```python
from build123d import *

# Parameters (mm, degrees)
ESQUISSE2_R             = 1.5
ENL_V_MAT_EXTRU_1_DEPTH = 21.928449536
ESQUISSE3_W             = 17.74823935
ESQUISSE3_H             = 7.774498086
ENL_V_MAT_EXTRU_2_DEPTH = 20.052558883
CONG_1_R                = 1


with BuildPart() as part:
    # Esquisse1 → R_volution1 (revolve)
    with BuildSketch(Plane.XY, mode=Mode.PRIVATE) as r_volution1_sk:
        Polygon((4, 0), (4, 15), (5, 15), (5, 4), (11, 4), (11, 1), (5, 1), (5, 0), align=None)
    revolve(r_volution1_sk.sketch.rotate(Axis((0, 0, 0), (0, 1, 0)), 90), axis=Axis((0, 0, 0), (0, 1, 0)))

    # Esquisse2 → Enl_v. mat.-Extru.1 (cut, through all)
    with BuildSketch(Plane.XZ.offset(-1)):
        with Locations(Location((7.778174593, 0, 0), (0, 0, 270))):
            Circle(ESQUISSE2_R)
        with Locations(Location((0, -7.778174593, 0), (0, 0, 270))):
            Circle(ESQUISSE2_R)
        with Locations(Location((-7.778174593, 0, 0), (0, 0, 270))):
            Circle(ESQUISSE2_R)
        with Locations(Location((0, 7.778174593, 0), (0, 0, 270))):
            Circle(ESQUISSE2_R)
    extrude(amount=-ENL_V_MAT_EXTRU_1_DEPTH, mode=Mode.SUBTRACT)

    # Esquisse3 → Enl_v. mat.-Extru.2 (cut, through all)
    with BuildSketch(Plane(origin=(0, 4, 0), x_dir=(1, 0, 0), z_dir=(0, 1, 0))):
        with Locations((0, 10.387249043)):
            Rectangle(ESQUISSE3_W, ESQUISSE3_H)
    extrude(amount=-ENL_V_MAT_EXTRU_2_DEPTH, mode=Mode.SUBTRACT)

    # Cong_1
    # the kernel refuses this fillet: 1 mm, written as the material it takes off along each edge
    with BuildSketch(Plane(origin=(11.374119675, 1, -6.5), x_dir=(0, 0, 1), z_dir=(-1, 0, 0)), Plane(origin=(1.714971523, 1, -6.5), x_dir=(0, 0, 1), z_dir=(-1, 0, 0))) as cong_1_piece_1:
        with BuildLine():
            CenterArc((CONG_1_R, CONG_1_R), CONG_1_R, 180, 90)
            Line((0, CONG_1_R), (0, 0))
            Line((0, 0), (CONG_1_R, 0))
        make_face()
    extrude(amount=13.089091198, mode=Mode.SUBTRACT)
    with BuildSketch(Plane(origin=(1.714971523, 4, -6.5), x_dir=(0, 0, 1), z_dir=(-1, 0, 0)), Plane(origin=(11.374119675, 4, -6.5), x_dir=(0, 0, 1), z_dir=(-1, 0, 0))) as cong_1_piece_2:
        with BuildLine():
            CenterArc((CONG_1_R, -CONG_1_R), CONG_1_R, 90, 90)
            Line((0, -CONG_1_R), (0, 0))
            Line((0, 0), (CONG_1_R, 0))
        make_face()
    extrude(amount=13.089091198, mode=Mode.SUBTRACT)


solid = part.part
```
The listing builds one solid part. Answer for the finished solid, in the listing's coordinates (mm). A direction names the side the tool comes from. Round coordinates to 2 decimals unless told otherwise and drop trailing zeros. Loops run counter-clockwise (first coordinate to the right, second up) from the corner with the lowest first, then second, coordinate; pieces in that order, holes last. Notation, with made-up numbers: (25.25, 8) - (70.25, 8) arc R18 ccw to (70.25, 33) - close; hole circle Ø3 at (40.25, 63.5). An arc over 180 degrees is marked (long way). Use one line per item in the form item = value. Start each with the question number.
1. A tool of negligible diameter and unlimited length cuts with its end or side. For faces 1 (the face through (-4.9, 2.5, -6.5)), 2 (the face through (0, 9, 5)), from which of +Z, -Z, +X, -X, +Y, -Y can it reach the whole face along a straight path? Write none if from no direction.
2. The part is cut by section D-D on z = 9. Determine the outline of the cut face in (x, y), then the cut area to 3 significant figures.
3. The part is cut by section A-A on z = 0. Determine the outline of the cut face in (x, y).
4. The part is cut by section C-C on y = 11.5. Determine the outline of the cut face in (x, z).
5. Given pin 1 Ø2 at (y, z) = (5.5, 0) entering from +X; pin 2 Ø5 at (x, z) = (-7.78, 0) entering from -Y; pin 3 Ø1.5 at (x, y) = (-6, 11.5) entering from -Z; pin 4 Ø2 at (x, z) = (7.5, -4) entering from +Y, each flat-ended and moving along its own axis, determine where each tip first touches the part or whether it passes through.
6. Consider line 1 (X direction, y = 2.85, z = 0); line 2 (Y direction, x = 1, z = 5.75); line 3 (X direction, y = 13.5, z = 3). Determine where each line is inside the solid, lowest interval first. Write a range as [from, to].
7. For a pull along X with two mould halves and no side action, classify faces 3 (the face through (0.1, 3.8, -6.1)), 4 (the face through (0.451, 2.479, 6.347)), 5 (the face through (-0.22, 0.493, 4.995)) as pulls with the +X half, pulls with the -X half, needs draft (parallel to the pull), parting line crosses it, or undercut.
8. The part is cut by section B-B on x = 3.5. Determine the outline of the cut face in (y, z).
Geometry check:
q1.face_1 = -Z, +X, -X, +Y, -Y
q1.face_2 = +Y
q2.outline = (-6.32, 1) - (-0.87, 1) - (-0.87, 4) - (-6.32, 4) - close; (0.87, 1) - (6.32, 1) - (6.32, 4) - (0.87, 4) - close
q2.area = 32.7 mm^2
q3.outline = (-11, 1) - (-9.28, 1) - (-9.28, 4) - (-11, 4) - close; (-6.28, 1) - (-5, 1) - (-5, 0) - (-4, 0) - (-4, 15) - (-5, 15) - (-5, 4) - (-6.28, 4) - close; (4, 0) - (5, 0) - (5, 1) - (6.28, 1) - (6.28, 4) - (5, 4) - (5, 15) - (4, 15) - close; (9.28, 1) - (11, 1) - (11, 4) - (9.28, 4) - close
q4.outline = circle Ø10 at (0, 0); hole circle Ø8 at (0, 0)
q5.pin_1 = 5
q5.pin_2 = 1
q5.pin_3 = through
q5.pin_4 = 4
q6.line_1 = [-11, -9.28], [-6.28, -4], [4, 6.28], [9.28, 11]
q6.line_2 = [1, 4]
q6.line_3 = [-4, -2.65], [2.65, 4]
q7.face_3 = needs draft
q7.face_4 = undercut
q7.face_5 = parting line crosses it
q8.outline = (0, -3.57) - (1, -3.57) - (1, -5.5) arc R1 ccw to (2, -6.5) - (3, -6.5) arc R1 ccw to (4, -5.5) - (4, -3.57) - (15, -3.57) - (15, -1.94) - (0, -1.94) - close; (0, 1.94) - (15, 1.94) - (15, 3.57) - (4, 3.57) - (4, 10.43) - (1, 10.43) - (1, 3.57) - (0, 3.57) - close
